Autodesk Inventor part; units mm, degrees
ref_plane "YZ Plane" through (0, 0, 0) normal (1, 0, 0) x (0, 1, 0)
ref_plane "XZ Plane" through (0, 0, 0) normal (0, 1, 0) x (-1, 0, 0)
ref_plane "XY Plane" through (0, 0, 0) normal (0, 0, 1) x (1, 0, 0)
sketch "Sketch1" plane through (0, 0, 0) normal (0, 1, 0) x (-1, 0, 0)
  line L0 (0, 0) -> (0, 42.5039)
  line L1 (17, 42.5039) -> (20, 42.5039)
  line L2 (0, 42.5039) -> (17, 42.5039) construction
  line L3 (20, 42.5039) -> (22.85, 36.6194)
  line L4 (22.85, 20.25) -> (26.9, 20.25)
  line L5 (26.9, 20.25) -> (26.9, 4.05)
  line L6 (26.9, 4.05) -> (22.4, 4.05)
  line L7 (22.4, 4.05) -> (22.4, 0)
  line L8 (22.4, 0) -> (20.15, 0)
  line L9 (20.15, 0) -> (20.15, 6.3)
  line L10 (20.15, 6.3) -> (24.65, 6.3)
  line L11 (24.65, 6.3) -> (24.65, 18)
  line L12 (24.65, 18) -> (20.15, 18)
  line L13 (20.15, 18) -> (20.15, 36)
  line L14 (20.15, 36) -> (17, 42.5039)
  line L15 (20.15, 0) -> (0, 0) construction
  line L16 (22.85, 36.6194) -> (22.85, 20.25)
  line L17 (0, 42.5039) -> (0, 74.5039) construction
  line L18 (0, 74.5039) -> (-32, 74.5039) construction
  line L19 (-32, 74.5039) -> (-74.5039, 74.5039) construction
  line L20 (-74.5039, 74.5039) -> (-74.5039, 94.6539) construction
  line L21 (-74.5039, 94.6539) -> (-74.5039, 96.9039)
  line L22 (-74.5039, 96.9039) -> (-70.4539, 96.9039)
  line L23 (-70.4539, 96.9039) -> (-70.4539, 101.4039)
  line L24 (-70.4539, 101.4039) -> (-54.2539, 101.4039)
  line L25 (-54.2539, 101.4039) -> (-54.2539, 97.3539)
  line L26 (-54.2539, 97.3539) -> (-37.8845, 97.3539)
  line L27 (-37.8845, 97.3539) -> (-32, 94.5039)
  line L28 (-32, 94.5039) -> (-32, 91.5039)
  line L29 (-32, 91.5039) -> (-38.5039, 94.6539)
  line L30 (-38.5039, 94.6539) -> (-56.5039, 94.6539)
  line L31 (-56.5039, 94.6539) -> (-56.5039, 99.1539)
  line L32 (-56.5039, 99.1539) -> (-68.2039, 99.1539)
  line L33 (-68.2039, 99.1539) -> (-68.2039, 94.6539)
  line L34 (-68.2039, 94.6539) -> (-74.5039, 94.6539)
  line L35 (-32, 91.5039) -> (-32, 74.5039) construction
  line L36 (20.15, 36) -> (0, 36) construction
  line L37 (-38.5039, 94.6539) -> (-38.5039, 74.5039) construction
  dimension "d0" = 2.25
  dimension "d1" = 2.25
  dimension "d2" = 2.25
  dimension "d4" = 2.7
  dimension "d5" = 2.25
  dimension "d6" = 6.75
  dimension "d7" = 40.3
  dimension "d8" = 18
  dimension "d9" = 18
  dimension "d11" = 6.3
  dimension "d12" = 40
  dimension "d13" = 3
  dimension "d14" = 2.7
  dimension "d17" = 40.3
  dimension "d18" = 2.25
  dimension "d19" = 2.25
  dimension "d20" = 2.25
  dimension "d21" = 2.25
  dimension "d22" = 4.5
  dimension "d23" = 2.7
  dimension "d24" = 3
  dimension "d25" = 40
  dimension "d26" = 6.3
  dimension "d27" = 18
  dimension "d28" = 18
  dimension "d29" = 32
  dimension "d30" = 32
  dimension "d31" = 2.7
revolve "Revolution1" add sketch "Sketch1" angle 360 about axis through (0, 0, 0) along (0, 0, 1) contours L1 L3 L16 L4 L5 L6 L7 L8 L9 L10 L11 L12 L13 L14
sketch "Sketch2" plane through (0, 0, 42.5039) normal (0, 0, 1) x (1, 0, 0)
  circle A0 centre (0, 0) radius 20
  circle A1 centre (0, 0) radius 20
  circle A2 centre (0, 0) radius 17
  circle A3 centre (0, 0) radius 17
sketch "Sketch3" plane through (0, 0, 0) normal (0, 1, 0) x (-1, 0, 0)
  line L0 (-20, 42.5039) -> (20, 42.5039)
  line L1 (0, 42.5039) -> (0, 74.5039) construction
  line L2 (0, 74.5039) -> (-32, 74.5039) construction
  arc A0 (0, 42.5039) -> (-32, 74.5039) centre (-32, 42.5039) ccw
  dimension "d15" = 32
  dimension "d16" = 32
sweep "Sweep1" add profiles "Sketch2" path "Sketch3" path curves A0
revolve "Revolution2" add sketch "Sketch1" angle 360 about axis through (32, 0, 74.5039) along (1, 0, 0) contours L21 L22 L23 L24 L25 L26 L27 L28 L29 L30 L31 L32 L33 L34
equation "\"d0\" = e3"
equation "\"d1\" = e3"
equation "\"d2\" = e3"
equation "\"d4\" = e2"
equation "\"d5\" = e3"
equation "\"d6\" = 3 * e3"
equation "\"d7\" = Ds"
equation "\"d8\" = C1"
equation "\"d9\" = A"
equation "\"d11\" = 0.35 * C1"
equation "\"d12\" = De"
equation "\"d13\" = e"
equation "\"d14\" = e2"
equation "\"d17\" = Ds"
equation "\"d18\" = e3"
equation "\"d19\" = e3"
equation "\"d20\" = e3"
equation "\"d21\" = e3"
equation "\"d22\" = 2 * e3"
equation "\"d23\" = e2"
equation "\"d24\" = e"
equation "\"d25\" = De"
equation "\"d26\" = 0.35 * C1"
equation "\"d27\" = C1"
equation "\"d28\" = A"
equation "\"d29\" = z"
equation "\"d30\" = z"
equation "\"d31\" = e2"
equation "\"d15\" = z"
equation "\"d16\" = z"
equation "\"z\" = 32"
equation "\"De\" = 40"
equation "\"e\" = 3"
equation "\"Ds\" = 40.3"
equation "\"e2\" = 0.9 * e"
equation "\"C1\" = 18"
equation "\"e3\" = 0.75 * e"
equation "\"A\" = 18"
equation "\"Size_Designation\" = 1.2345"
properties part number "ISO 3633 Изгиб 90 с раструбом только для соединений с эластомерными уплотнительными кольцами DN40" material "ПВХ, непластифицированный"
CAD build for the part. Positions are in the model's coordinates, mm. A direction names the side the tool comes from. Coordinates: 2 decimals unless noted, no trailing zeros. Write each loop counter-clockwise with the first axis right and the second up, starting at its lowest first coordinate (ties: lowest second). Pieces come first, ordered by that corner, then holes. Notation, with made-up numbers: (32.25, -0.5) - (41.25, -0.5) arc R24 ccw to (41.25, 35.5) - close; hole circle Ø11 at (74, 55.25). An arc over 180 degrees is marked (long way). Use a Markdown table: item, result. Add a question column.
Item 1: Band-saw the part on B-B, the plane x = 65. Give the cut face in (y, z), and give its area (3 significant figures).
Item 2: Flat gauge pins, fed straight in: pin 1 (16 mm diameter, centred on y = -2.5, z = 75, fed in from -X); pin 2 (6 mm diameter, centred on x = 62, z = 42, fed in from -Y); pin 3 (24 mm diameter, centred on x = 0, y = 0, fed in from -Z); pin 4 (8 mm diameter, centred on y = -15, z = 34, fed in from -X). Where does each tip first touch, or does it go through?
Item 3: Drill centre lines: L1, parallel to X at y = 0, z = 32.25; L2, parallel to X at y = 0, z = 14; L3, parallel to Z at x = 66, y = 0. Where is each one in solid material? Low to high. Write a range as from..to.
Item 4: Mould opens along X. For faces 1 (the face through (68.204, 0, 54)), 2 (the face through (16.841, 15.443, 28.32)), 3 (the face through (71.398, 7.718, 93.117)) say: pulls with the +X half, pulls with the -X half, needs draft (parallel to the pull), parting line crosses it, or undercut.
Item 5: Band-saw the part on A-A, the plane z = 14. Give the cut face in (x, y), and give its area (3 significant figures).
Item 6: 3-axis set-ups, long thin cutter, end or side, ignore diameter. For faces 4 (the face through (-18.613, 7.718, 27.126)), 5 (the face through (47.63, 7.718, 93.117)), 6 (the face through (20.02, -3.42, 0)), 7 (the face through (54.254, 20, 62)): which of +Z, -Z, +X, -X, +Y, -Y reach the whole face in a straight line?
Numbers:
| question | item | result |
|---|---|---|
| 1 | outline | circle Ø53.8 at (0, 74.5); hole circle Ø49.3 at (0, 74.5) |
| 1 | area | 364 mm2 |
| 2 | pin 1 | x = -13.77 |
| 2 | pin 2 | through |
| 2 | pin 3 | z = 64.07 |
| 2 | pin 4 | x = -20.03 |
| 3 | L1 | -22.85..-20.15, 20.15..22.85 |
| 3 | L2 | -26.9..-24.65, 24.65..26.9 |
| 3 | L3 | 47.6..49.85, 99.15..101.4 |
| 4 | face 1 | undercut |
| 4 | face 2 | parting line crosses it |
| 4 | face 3 | needs draft |
| 5 | outline | circle Ø53.8 at (0, 0); hole circle Ø49.3 at (0, 0) |
| 5 | area | 364 mm2 |
| 6 | face 4 | -Z |
| 6 | face 5 | +X |
| 6 | face 6 | -Z, +X, -X, +Y, -Y |
| 6 | face 7 | none |
